from build123d import *

# Parameters (mm, degrees)
BOSS_EXTRUDE1_DEPTH = 60
SKETCH2_R           = 2.5
CUT_EXTRUDE1_DEPTH  = 18.65
FILLET1_R           = 3


with BuildPart() as part:
    # Sketch1 → Boss-Extrude1 (new body)
    with BuildSketch(Plane.XY):
        Polygon((0, 0), (25, 0), (25, 11.65), (69, 11.65), (69, 0), (94, 0), (94, 10), (79, 10), (79, 17.65), (15, 17.65), (15, 10), (0, 10), align=None)
    extrude(amount=BOSS_EXTRUDE1_DEPTH)

    # Sketch2 → Cut-Extrude1 (cut, through all)
    with BuildSketch(Plane(origin=(0, 17.65, 0), x_dir=(1, 0, 0), z_dir=(0, 1, 0))):
        with Locations((7, -7.5)):
            Circle(SKETCH2_R)
        with Locations((7, -51.5)):
            Circle(SKETCH2_R)
        with Locations((87, -7.5)):
            Circle(SKETCH2_R)
        with Locations((87, -51.5)):
            Circle(SKETCH2_R)
        with BuildLine():
            Line((29.75, -36), (29.75, -55))
            ThreePointArc((29.75, -55), (31.5, -56.75), (33.25, -55))
            Line((33.25, -55), (33.25, -36))
            ThreePointArc((33.25, -36), (31.5, -34.25), (29.75, -36))
        make_face()
        with BuildLine():
            Line((29.75, -24), (29.75, -5))
            ThreePointArc((29.75, -5), (31.5, -3.25), (33.25, -5))
            Line((33.25, -5), (33.25, -24))
            ThreePointArc((33.25, -24), (31.5, -25.75), (29.75, -24))
        make_face()
        with BuildLine():
            Line((60.75, -5), (60.75, -24))
            ThreePointArc((60.75, -24), (62.5, -25.75), (64.25, -24))
            Line((64.25, -24), (64.25, -5))
            ThreePointArc((64.25, -5), (62.5, -3.25), (60.75, -5))
        make_face()
        with BuildLine():
            Line((60.75, -36), (60.75, -55))
            ThreePointArc((60.75, -55), (62.5, -56.75), (64.25, -55))
            Line((64.25, -55), (64.25, -36))
            ThreePointArc((64.25, -36), (62.5, -34.25), (60.75, -36))
        make_face()
        with BuildLine():
            Line((35.5, -20.5), (35.5, -39.5))
            ThreePointArc((35.5, -39.5), (47, -51), (58.5, -39.5))
            Line((58.5, -39.5), (58.5, -20.5))
            ThreePointArc((58.5, -20.5), (47, -9), (35.5, -20.5))
        make_face()
    extrude(amount=-CUT_EXTRUDE1_DEPTH, mode=Mode.SUBTRACT)

    # Fillet1
    fillet1_edges = [part.edges().sort_by_distance(p)[0] for p in [
        (0, 10, 30),
        (15, 17.65, 30),
        (79, 17.65, 30),
        (94, 10, 30),
    ]]
    fillet(fillet1_edges, radius=FILLET1_R)


solid = part.part
Source: CAD feature listing. Evaluate the final solid. Frame: model axes, mm. A direction names the side the tool comes from. Give positions to 0.01 mm unless a question says otherwise; leave off trailing zeros. Order: outer loops, then holes, each group sorted by start corner. A loop starts at its lowest first (then second) coordinate and runs counter-clockwise, first axis right, second up. Notation, with made-up numbers: (-8.5, 31.25) -> (22.5, 31.25) arc R27 cw to (22.5, 61.25) -> close; hole circle Ø2 at (-31.75, -38). An arc over 180 degrees is marked (long way). Write item = value, one per line.
Q1. Cut plane A-A, the plane z = 7.5. State how many separate pieces and enclosed holes the cut face has, and give its area (3 significant figures).
Data:
separate_pieces = 5
enclosed_holes = 0
area = 767 mm^2
Q2. Set-up query: faces 5 (the face through (79, 12, 30)), 6 (the face through (25, 6, 30)), 7 (the face through (31.54, 14.69, 25.75)). Return all of +Z, -Z, +X, -X, +Y, -Y with unobstructed straight access to the full face (end or side cutting, diameter ignored); none if empty.
Data:
face_5 = +Z, -Z, +X, +Y
face_6 = +Z, -Z, -Y
face_7 = +Y, -Y
Q3. Material intervals for line 1 (X direction, y = 3.75, z = 51.5); line 2 (Z direction, x = 7, y = 3); line 3 (X direction, y = 4.25, z = 11.5), sorted ascending. Write a range as from..to.
Data:
line_1 = 0..4.5, 9.5..25, 69..84.5, 89.5..94
line_2 = 0..5, 10..49, 54..60
line_3 = 0..25, 69..94
Q4. Cut plane B-B, the plane y = 13.5. Output: boundary loops of the cut face in (x, z).
Data:
outline = (15, 0) -> (79, 0) -> (79, 60) -> (15, 60) -> close; hole (29.75, 5) arc R1.75 ccw to (33.25, 5) -> (33.25, 24) arc R1.75 ccw to (29.75, 24) -> close; hole (29.75, 36) arc R1.75 ccw to (33.25, 36) -> (33.25, 55) arc R1.75 ccw to (29.75, 55) -> close; hole (35.5, 20.5) arc R11.5 ccw to (58.5, 20.5) -> (58.5, 39.5) arc R11.5 ccw to (35.5, 39.5) -> close; hole (60.75, 5) arc R1.75 ccw to (64.25, 5) -> (64.25, 24) arc R1.75 ccw to (60.75, 24) -> close; hole (60.75, 36) arc R1.75 ccw to (64.25, 36) -> (64.25, 55) arc R1.75 ccw to (60.75, 55) -> close
Q5. Cut plane D-D, the plane z = 13.5. Output: boundary loops of the cut face in (x, y), and give its area (3 significant figures).
Data:
outline = (0, 0) -> (25, 0) -> (25, 11.65) -> (29.75, 11.65) -> (29.75, 17.65) -> (18, 17.65) arc R3 ccw to (15, 14.65) -> (15, 10) -> (3, 10) arc R3 ccw to (0, 7) -> close; (33.25, 11.65) -> (37.88, 11.65) -> (37.88, 17.65) -> (33.25, 17.65) -> close; (56.12, 11.65) -> (60.75, 11.65) -> (60.75, 17.65) -> (56.12, 17.65) -> close; (64.25, 11.65) -> (69, 11.65) -> (69, 0) -> (94, 0) -> (94, 7) arc R3 ccw to (91, 10) -> (79, 10) -> (79, 14.65) arc R3 ccw to (76, 17.65) -> (64.25, 17.65) -> close
area = 758 mm^2
Q6. Pin query (flat end, axial travel): pin 1 (3 mm diameter, centred on y = 15, z = 34.5, fed in from -X); pin 2 (1.8 mm diameter, centred on y = 15.5, z = 42.5, fed in from +X); pin 3 (3.5 mm diameter, centred on x = 6.5, z = 30, fed in from +Y). Return the tip coordinate at first contact, or that it passes through.
Data:
pin_1 = 15
pin_2 = 79
pin_3 = 10
Q7. Cut plane C-C, the plane x = 62.5. Output: boundary loops of the cut face in (y, z).
Data:
outline = (11.65, 0) -> (17.65, 0) -> (17.65, 3.25) -> (11.65, 3.25) -> close; (11.65, 25.75) -> (17.65, 25.75) -> (17.65, 34.25) -> (11.65, 34.25) -> close; (11.65, 56.75) -> (17.65, 56.75) -> (17.65, 60) -> (11.65, 60) -> close
Q8. Pull-direction query (X, two-part tool) for faces 1 (the face through (85, 5, 9)), 2 (the face through (0, 4, 30)), 3 (the face through (31.54, 14.69, 34.25)), 4 (the face through (9, 10, 30)); classes: released by +X, released by -X, zero draft, split by the parting line, or undercut.
Data:
face_1 = undercut
face_2 = released by -X
face_3 = undercut
face_4 = zero draft
